The model under review builds one solid part; all positions refer to its coordinate system, in mm. Face numbers are marked on the shaded views. Coordinates: 2 decimals unless noted, no trailing zeros. Loops run counter-clockwise (first coordinate to the right, second up) from the corner with the lowest first, then second, coordinate; pieces in that order, holes last. Notation, with made-up numbers: M 16.25,34 L 66.25,34 A20 cw 66.25,39 Z; hole C -28.5,15.5 d5. An arc over 180 degrees is marked long. Use one line per item in the form item = value.
```python
from build123d import *

# Parameters (mm, degrees)
SKETCH1_R           = 32
SKETCH1_R_2         = 1
BOSS_EXTRUDE1_DEPTH = 11
SKETCH7_R           = 7
SKETCH7_R_2         = 1
BOSS_EXTRUDE3_DEPTH = 11


with BuildPart() as part:
    # Sketch1 → Boss-Extrude1 (new body)
    with BuildSketch(Plane.XY):
        Circle(SKETCH1_R)
        Circle(SKETCH1_R_2, mode=Mode.SUBTRACT)
    extrude(amount=BOSS_EXTRUDE1_DEPTH)

    # Sketch4 → Cut-Revolve1 (revolve, cut)
    with BuildSketch(Plane(origin=(0, 0, 0), x_dir=(0, 0, -1), z_dir=(1, 0, 0)), mode=Mode.PRIVATE) as cut_revolve1_sk:
        Polygon((-2, 32), (-3, 30), (-8, 30), (-9, 32), align=None)
    revolve(cut_revolve1_sk.sketch.rotate(Axis((0, 0, 1000), (0, 0, -1)), 90), axis=Axis((0, 0, 1000), (0, 0, -1)), mode=Mode.SUBTRACT)

    # Sketch7 → Boss-Extrude3 (add)
    with BuildSketch(Plane.XY.offset(11)):
        Circle(SKETCH7_R)
        Circle(SKETCH7_R_2, mode=Mode.SUBTRACT)
    extrude(amount=BOSS_EXTRUDE3_DEPTH)

    # Sketch8 → Cut-Revolve3 (revolve, cut)
    with BuildSketch(Plane(origin=(0, 0, 0), x_dir=(0, 0, -1), z_dir=(1, 0, 0)), mode=Mode.PRIVATE) as cut_revolve3_sk:
        Polygon((-20, 7), (-13, 7), (-14, 5), (-19, 5), align=None)
    revolve(cut_revolve3_sk.sketch.rotate(Axis((0, 0, 1000), (0, 0, -1)), 90), axis=Axis((0, 0, 1000), (0, 0, -1)), mode=Mode.SUBTRACT)


solid = part.part
```
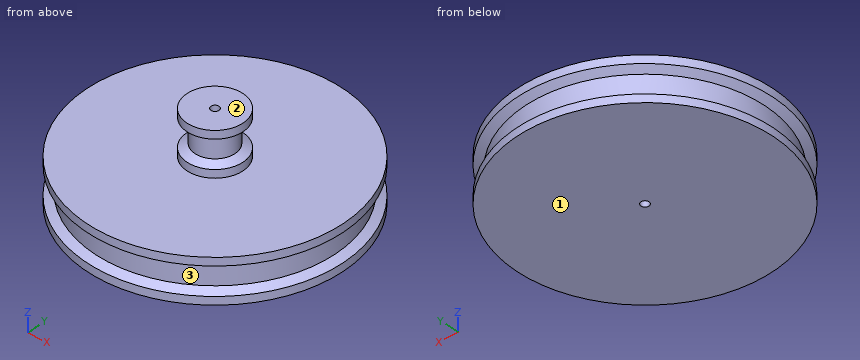
1. Wall thickness on line 1 along Y through (x, z) = (0, 17.25); line 2 along Z through (x, y) = (-16, 2); line 3 along Y through (x, z) = (0, 13.5): over which ranges is each line inside the solid? List them lowest first. Write a range as from..to.
Response values:
line_1 = -5..-1, 1..5
line_2 = 0..11
line_3 = -6..-1, 1..6
2. Insertion check: P1, Ø8, axis at y = 14.5, z = 13, coming from the -X side; P2, Ø1.5, axis at x = 20, y = 9, coming from the +Z side; P3, Ø1.8, axis at x = 0, y = 0, coming from the -Z side; P4, Ø5, axis at x = -0.5, y = 15, coming from the -Z side. Each pin has a flat end and moves straight along its axis. Give the tip position at first contact, or say it passes through.
Response values:
P1 = -30.04
P2 = 11
P3 = through
P4 = 0
3. Add section C-C (z = 15.5). State the section outline as (x, y) points, then the cut area to 3 significant figures.
Response values:
outline = C 0,0 d10; hole C 0,0 d2
area = 75.4 mm^2
4. The part is to be moulded in two halves that separate along Z. For the marked faces 1, 2 and 3, say which applies: pulls with the +Z half, pulls with the -Z half, needs draft (parallel to the pull), parting line crosses it, or undercut.
Response values:
face_1 = pulls with the -Z half
face_2 = pulls with the +Z half
face_3 = undercut
5. Add section A-A (x = 0). State the section outline as (y, z) points.
Response values:
outline = M -32,0 L -1,0 L -1,22 L -7,22 L -7,20 L -5,19 L -5,14 L -7,13 L -7,11 L -32,11 L -32,9 L -30,8 L -30,3 L -32,2 Z; M 1,0 L 32,0 L 32,2 L 30,3 L 30,8 L 32,9 L 32,11 L 7,11 L 7,13 L 5,14 L 5,19 L 7,20 L 7,22 L 1,22 Z
